The listing builds one solid part. Answer for the finished solid, in the listing's coordinates (mm). Face numbers are marked on the shaded views. A direction names the side the tool comes from. Round coordinates to 2 decimals unless told otherwise and drop trailing zeros. Loops run counter-clockwise (first coordinate to the right, second up) from the corner with the lowest first, then second, coordinate; pieces in that order, holes last. Notation, with made-up numbers: (27.25, 6) - (72.25, 6) arc R22 ccw to (72.25, 14) - close; hole circle Ø7 at (-22, 83.25). An arc over 180 degrees is marked (long way). Write item = value, one per line. Start each with the question number.
1) For a pull along X with two mould halves and no side action, classify the marked faces 1 and 2 as released by +X, released by -X, zero draft, split by the parting line, or undercut.
2) Section D-D, the plane y = 22 is taken. Determine the outline of the cut face in (x, z), and give its area (3 significant figures).
3) A tool of negligible diameter and unlimited length cuts with its end or side. For the marked faces 3 and 4, from which of +Z, -Z, +X, -X, +Y, -Y can it reach the whole face along a straight path? Write none if from no direction.
4) Straight lines are drawn through the part: line 1 along Z through (x, y) = (13.5, 21.5); line 2 along X through (y, z) = (34, 5); line 3 along X through (y, z) = (38, 4). For each, find the intervals that lie inside material, in ascending order.
5) Section C-C, the plane z = 15 is taken. Determine the outline of the cut face in (x, y).
6) Section B-B, the plane y = 37 is taken. Determine the outline of the cut face in (x, z).
7) Section A-A, the plane x = 45 is taken. Determine the outline of the cut face in (y, z), and give its area (3 significant figures).
8) Given pin 1 Ø3 at (x, y) = (58, 30) entering from +Z; pin 2 Ø8 at (x, z) = (53.5, 9.5) entering from -Y, each flat-ended and moving along its own axis, determine where each tip first touches the part or whether it passes through.
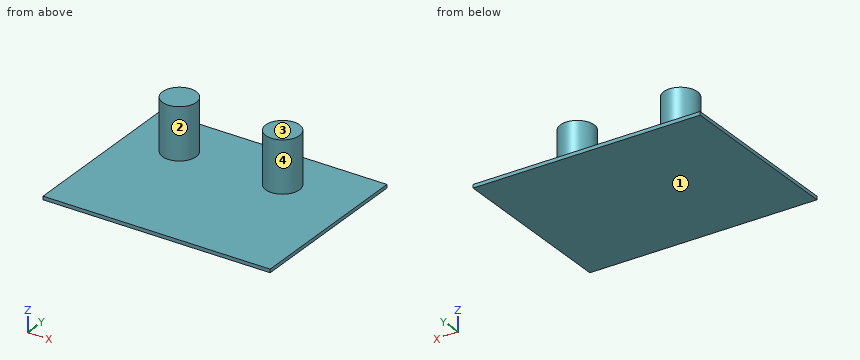
from build123d import *

# Parameters (mm, degrees)
ESQUISSE2_W        = 66
ESQUISSE2_H        = 51
ESQUISSE2_R        = 6
ESQUISSE2_W_2      = 20
ESQUISSE2_H_2      = 41
ESQUISSE2_R_2      = 4.9
BOSS_EXTRU_1_DEPTH = 1
ESQUISSE4_R        = 4.9
BOSS_EXTRU_2_DEPTH = 15


with BuildPart() as part:
    # Esquisse2 → Boss.-Extru.1 (new body)
    # profile 1 of 5: a face of its own
    with BuildSketch(Plane.XY):
        with Locations((33, 25.5)):
            Rectangle(ESQUISSE2_W, ESQUISSE2_H)
        with Locations((55, 37)):
            Circle(ESQUISSE2_R, mode=Mode.SUBTRACT)
        with Locations((15, 25.5)):
            Rectangle(ESQUISSE2_W_2, ESQUISSE2_H_2, mode=Mode.SUBTRACT)
    # profile 2 of 5: a face of its own
    with BuildSketch(Plane.XY):
        with Locations((15, 25.5)):
            Rectangle(ESQUISSE2_W_2, ESQUISSE2_H_2)
        with Locations((15, 37)):
            Circle(ESQUISSE2_R_2, mode=Mode.SUBTRACT)
    # profile 3 of 5: a face of its own
    with BuildSketch(Plane.XY):
        with Locations((15, 37)):
            Circle(ESQUISSE2_R_2)
    # profile 4 of 5: a face of its own
    with BuildSketch(Plane.XY):
        with Locations((55, 37)):
            Circle(ESQUISSE2_R)
        with Locations((55, 37)):
            Circle(ESQUISSE2_R_2, mode=Mode.SUBTRACT)
    # profile 5 of 5: a face of its own
    with BuildSketch(Plane.XY):
        with Locations((55, 37)):
            Circle(ESQUISSE2_R_2)
    extrude(amount=BOSS_EXTRU_1_DEPTH)

    # Esquisse4 → Boss.-Extru.2 (add)
    with BuildSketch(Plane.XY.offset(1)):
        with Locations((15, 37)):
            Circle(ESQUISSE4_R)
        with Locations((45, 37)):
            Circle(ESQUISSE4_R)
    extrude(amount=BOSS_EXTRU_2_DEPTH)


solid = part.part
Geometry check:
q1.face_1 = zero draft
q1.face_2 = undercut
q2.outline = (0, 0) - (66, 0) - (66, 1) - (0, 1) - close
q2.area = 66.0 mm2
q3.face_3 = +Z, +X, -X, +Y, -Y
q3.face_4 = +Z
q4.line_1 = 0 to 1
q4.line_2 = 11.13 to 18.87, 41.13 to 48.87
q4.line_3 = 10.2 to 19.8, 40.2 to 49.8
q5.outline = circle Ø9.8 at (15, 37); circle Ø9.8 at (45, 37)
q6.outline = (0, 0) - (66, 0) - (66, 1) - (49.9, 1) - (49.9, 16) - (40.1, 16) - (40.1, 1) - (19.9, 1) - (19.9, 16) - (10.1, 16) - (10.1, 1) - (0, 1) - close
q7.outline = (0, 0) - (51, 0) - (51, 1) - (41.9, 1) - (41.9, 16) - (32.1, 16) - (32.1, 1) - (0, 1) - close
q7.area = 198 mm2
q8.pin_1 = 1
q8.pin_2 = 35.06
